The model under review builds one solid part; all positions refer to its coordinate system, in mm. Give positions to 0.01 mm unless a question says otherwise; leave off trailing zeros. Loops run counter-clockwise (first coordinate to the right, second up) from the corner with the lowest first, then second, coordinate; pieces in that order, holes last. Notation, with made-up numbers: M -36,59.25 L 2,59.25 A18 ccw 2,85.25 Z; hole C 36.25,35.25 d9. An arc over 180 degrees is marked long. One line per item, written item: value. Start each with the question number.
Q1. Mouldability with a two-part tool opening along X and no side actions: class faces 1 (the face through (-121.735, -75.049, 0.781)), 2 (the face through (-150.073, -135.862, -0.084)), 3 (the face through (121.735, -75.049, 0.781)), 4 (the face through (150.073, -135.862, -0.084)) as released by +X, released by -X, zero draft, split by the parting line, or undercut.
Q2. We need section A-A on z = 0. Write out the cut boundary in (x, y).
Q3. We need section B-B on x = 25.5. Write out the cut boundary in (y, z), plus the area to 3 significant figures.
Q4. For pin 1 (1.5 mm diameter, centred on x = 108.5, z = 4.5, fed in from +Y); pin 2 (10 mm diameter, centred on x = -121, y = -67, fed in from -Z); pin 3 (3 mm diameter, centred on y = -81.5, z = 0, fed in from -X), all flat-tipped, find the tip position at first contact; note any pin that passes through.
Q5. To check wall thickness, follow line 1 along X through (y, z) = (-128.5, 0.75); line 2 along X through (y, z) = (-101, -1.75); line 3 along Y through (x, z) = (-18.5, 0). State the ranges of each line that lie inside material, in increasing order. Write a range as from..to.
```python
from build123d import *

# Parameters (mm, degrees)
SKETCH_1_R = 6


with BuildPart() as part:
    # По траектории1: sweep along a path in Эскиз2
    with BuildLine(Plane.XY) as sweep_1_path:
        Line((0, -6), (60.56624327, -6))
        ThreePointArc((60.56624327, -6), (73.06624327, -9.349364905), (82.216878365, -18.5))
        Line((82.216878365, -18.5), (150, -135.903810568))
    # Эскиз1 → По траектории1 (sweep)
    with BuildSketch(Plane(origin=(0, 0, 0), x_dir=(0, 0, -1), z_dir=(1, 0, 0))):
        with Locations((0, -6)):
            Circle(SKETCH_1_R)
    sweep_1 = sweep(path=sweep_1_path.line)

    # Зеркальное отражение1: По траектории1 across plane
    add(sweep_1.mirror(Plane(origin=(0, -6, 0), x_dir=(0, 0, 1), z_dir=(1, 0, 0))))


solid = part.part
```
Solved:
1. face 1: undercut
1. face 2: released by -X
1. face 3: undercut
1. face 4: released by +X
2. outline: M -155.2,-132.9 L -144.8,-138.9 L -77.02,-21.5 A19 cw -60.57,-12 L 60.57,-12 A19 cw 77.02,-21.5 L 144.8,-138.9 L 155.2,-132.9 L 87.41,-15.5 A31 ccw 60.57,0 L -60.57,0 A31 ccw -87.41,-15.5 Z
3. outline: C -6,0 d12
3. area: 113 mm2
4. pin 1: y = -54.11
4. pin 2: z = -4.15
4. pin 3: x = -126.38
5. line 1: -152.6..-138.85, 138.85..152.6
5. line 2: -136.48..-123.22, 123.22..136.48
5. line 3: -12..0
